from build123d import *

# Parameters (mm, degrees)
SKETCH_1_W           = 89.43
SKETCH_1_H           = 60
EXTRUDE_2_DEPTH      = 50
EXTRUDE_START        = -50
EXTRUDE_3_OUTLINE_W  = 85.42
EXTRUDE_3_OUTLINE_H  = 56
EXTRUDE_3_DEPTH      = 50
SKETCH_3_W           = 89.43
SKETCH_3_H           = 60
EXTRUDE_4_DEPTH      = 2
EXTRUDE_START_2      = -2
EXTRUDE_5_OUTLINE_W  = 73.44
EXTRUDE_5_OUTLINE_H  = 48.96
EXTRUDE_5_DEPTH      = 2
SKETCH_6_W           = 2
SKETCH_6_H           = 12
CUT_EXTRUDE_6_DEPTH  = 10
SKETCH_8_W           = 6
SKETCH_8_H           = 16
CUT_EXTRUDE_7_DEPTH  = 10
DRAFT_2_ANGLE        = 45
SKETCH_9_W           = 61
SKETCH_9_H           = 3
EXTRUDE_5_2_DEPTH    = 7
SKETCH_10_W          = 3
SKETCH_10_H          = 40
EXTRUDE_6_DEPTH      = 7
SKETCH_11_W          = 8
SKETCH_11_H          = 2
EXTRUDE_7_DEPTH      = 20
SKETCH_12_W          = 3
SKETCH_12_H          = 7
CUT_EXTRUDE_8_DEPTH  = 6
SKETCH_13_W          = 8
SKETCH_13_H          = 2
EXTRUDE_8_DEPTH      = 11
SKETCH_14_W          = 3
SKETCH_14_H          = 56
CUT_EXTRUDE_10_DEPTH = 11
SKETCH_15_W          = 87.425
SKETCH_15_H          = 2
CUT_EXTRUDE_11_DEPTH = 1
SKETCH_16_W          = 87.425
SKETCH_16_H          = 2
CUT_EXTRUDE_12_DEPTH = 1
SKETCH_17_R          = 3
CUT_EXTRUDE_13_DEPTH = 5.4
EXTRUDE_9_DEPTH      = 3.6
SKETCH_20_W          = 3
SKETCH_20_H          = 2
EXTRUDE_10_DEPTH     = 7
CUT_EXTRUDE_15_DEPTH = 7
SKETCH_22_W          = 32
SKETCH_22_H          = 58
CUT_EXTRUDE_16_DEPTH = 1
SKETCH_25_W          = 3
SKETCH_25_H          = 2
CUT_EXTRUDE_18_DEPTH = 2
SKETCH_27_W          = 4
SKETCH_27_H          = 2
CUT_EXTRUDE_19_DEPTH = 2
SKETCH_29_W          = 2.005
SKETCH_29_H          = 11.917011913
EXTRUDE_12_DEPTH     = 17
SKETCH_31_W          = 1.611039623
SKETCH_31_H          = 56
SKETCH_31_W_2        = 2
CUT_EXTRUDE_20_DEPTH = 48
SKETCH_34_W          = 8.005
SKETCH_34_H          = 34
EXTRUDE_13_DEPTH     = 2
SKETCH_35_W          = 8.005
SKETCH_35_H          = 3
EXTRUDE_14_DEPTH     = 8
SKETCH_36_R          = 3
CUT_EXTRUDE_21_DEPTH = 8
SKETCH_37_W          = 4
SKETCH_37_H          = 2
CUT_EXTRUDE_22_DEPTH = 5
SKETCH_38_W          = 10
SKETCH_38_H          = 3
CUT_EXTRUDE_23_DEPTH = 4.5
SKETCH_39_W          = 1.5
SKETCH_39_H          = 5
CUT_EXTRUDE_24_DEPTH = 20


# Read off the part's stored shape, not the designer's step: 切除-拉伸3, 切除-拉伸5
with BuildPart() as part:
    # 草图1 → 凸台-拉伸2 (new body)
    with BuildSketch(Plane.XY):
        Rectangle(SKETCH_1_W, SKETCH_1_H)
    extrude(amount=EXTRUDE_2_DEPTH)

    # 切除-拉伸3 outline → 切除-拉伸3 (cut)
    with BuildSketch(Plane.XY.offset(50).offset(EXTRUDE_START)):
        Rectangle(EXTRUDE_3_OUTLINE_W, EXTRUDE_3_OUTLINE_H)
    extrude(amount=EXTRUDE_3_DEPTH, mode=Mode.SUBTRACT)

    # 草图3 → 凸台-拉伸4 (add)
    with BuildSketch(Plane.XY.offset(50)):
        Rectangle(SKETCH_3_W, SKETCH_3_H)
    extrude(amount=-EXTRUDE_4_DEPTH)

    # Extrude 5 outline → Extrude 5 (cut)
    with BuildSketch(Plane.XY.offset(50).offset(EXTRUDE_START_2)):
        with Locations((-2.475, 0)):
            Rectangle(EXTRUDE_5_OUTLINE_W, EXTRUDE_5_OUTLINE_H)
    extrude(amount=EXTRUDE_5_DEPTH, mode=Mode.SUBTRACT)

    # 草图6 → 切除-拉伸6 (cut)
    with BuildSketch(Plane.ZY.offset(44.715)):
        with Locations((26.25, 14.9)):
            Rectangle(SKETCH_6_W, SKETCH_6_H)
    extrude(amount=-CUT_EXTRUDE_6_DEPTH, mode=Mode.SUBTRACT)

    # 草图8 → 切除-拉伸7 (cut)
    with BuildSketch(Plane.ZY.offset(44.715)):
        with Locations((26.25, 14.9)):
            Rectangle(SKETCH_8_W, SKETCH_8_H)
    extrude(amount=-CUT_EXTRUDE_7_DEPTH, mode=Mode.SUBTRACT)

    # 拔模2
    draft_2_faces = [part.faces().sort_by_distance(p)[0] for p in [
        (-43.7125, 22.9, 26.25),
        (-43.7125, 14.9, 23.25),
        (-43.7125, 6.9, 26.25),
        (-43.7125, 14.9, 29.25),
    ]]
    draft(draft_2_faces, Plane(origin=(-44.715, 30, 50), x_dir=(0, -1, 0), z_dir=(-1, 0, 0)), DRAFT_2_ANGLE)

    # 草图9 → Extrude 5 2 (add)
    with BuildSketch(Plane(origin=(0, -28, 0), x_dir=(1, 0, 0), z_dir=(0, 1, 0))):
        with Locations((-12.21, -38.5)):
            Rectangle(SKETCH_9_W, SKETCH_9_H)
    extrude(amount=EXTRUDE_5_2_DEPTH)

    # 草图10 → 凸台-拉伸6 (add)
    with BuildSketch(Plane(origin=(0, -28, 0), x_dir=(1, 0, 0), z_dir=(0, 1, 0))):
        with Locations((16.79, -20)):
            Rectangle(SKETCH_10_W, SKETCH_10_H)
    extrude(amount=EXTRUDE_6_DEPTH)

    # 草图11 → 凸台-拉伸7 (add)
    with BuildSketch(Plane(origin=(0, 0, 37), x_dir=(-1, 0, 0), z_dir=(0, 0, -1))):
        with Locations((-11.29, -22)):
            Rectangle(SKETCH_11_W, SKETCH_11_H)
        with Locations((38.71, -22)):
            Rectangle(SKETCH_11_W, SKETCH_11_H)
    extrude(amount=EXTRUDE_7_DEPTH)

    # 草图12 → 切除-拉伸8 (cut)
    with BuildSketch(Plane(origin=(0, 0, 0), x_dir=(-1, 0, 0), z_dir=(0, 0, -1))):
        with Locations((-16.79, -24.5)):
            Rectangle(SKETCH_12_W, SKETCH_12_H)
    extrude(amount=-CUT_EXTRUDE_8_DEPTH, mode=Mode.SUBTRACT)

    # 草图13 → 凸台-拉伸8 (add)
    with BuildSketch(Plane(origin=(0, 0, 17), x_dir=(-1, 0, 0), z_dir=(0, 0, -1))):
        with Locations((-11.29, -22)):
            Rectangle(SKETCH_13_W, SKETCH_13_H)
        with Locations((38.71, -22)):
            Rectangle(SKETCH_13_W, SKETCH_13_H)
    extrude(amount=EXTRUDE_8_DEPTH)

    # 草图14 → 切除-拉伸10 (cut)
    with BuildSketch(Plane(origin=(44.715, 0, 0), x_dir=(0, 0, -1), z_dir=(1, 0, 0))):
        with Locations((-1.5, 0)):
            Rectangle(SKETCH_14_W, SKETCH_14_H)
    extrude(amount=-CUT_EXTRUDE_10_DEPTH, mode=Mode.SUBTRACT)

    # 草图15 → 切除-拉伸11 (cut)
    with BuildSketch(Plane.XZ.offset(-28)):
        with Locations((1.0025, 2)):
            Rectangle(SKETCH_15_W, SKETCH_15_H)
    extrude(amount=-CUT_EXTRUDE_11_DEPTH, mode=Mode.SUBTRACT)

    # 草图16 → 切除-拉伸12 (cut)
    with BuildSketch(Plane(origin=(0, -28, 0), x_dir=(1, 0, 0), z_dir=(0, 1, 0))):
        with Locations((1.0025, -2)):
            Rectangle(SKETCH_16_W, SKETCH_16_H)
    extrude(amount=-CUT_EXTRUDE_12_DEPTH, mode=Mode.SUBTRACT)

    # 草图17 → 切除-拉伸13 (cut)
    with BuildSketch(Plane.ZY.offset(44.715)):
        with Locations(Location((11.4, 18, 0), (0, 0, 270))):
            Circle(SKETCH_17_R)
    extrude(amount=-CUT_EXTRUDE_13_DEPTH, mode=Mode.SUBTRACT)

    # 草图18 → 凸台-拉伸9 (add)
    with BuildSketch(Plane(origin=(0, -28, 0), x_dir=(1, 0, 0), z_dir=(0, 1, 0))):
        Polygon((18.29, -25), (18.29, -27), (40.29, -27), (40.29, -18), (38.29, -18), (38.29, -25), align=None)
    extrude(amount=EXTRUDE_9_DEPTH)

    # 草图20 → 凸台-拉伸10 (add)
    with BuildSketch(Plane(origin=(0, 0, 25), x_dir=(-1, 0, 0), z_dir=(0, 0, -1))):
        with Locations((-36.79, -25.4)):
            Rectangle(SKETCH_20_W, SKETCH_20_H)
        with Locations((-19.79, -25.4)):
            Rectangle(SKETCH_20_W, SKETCH_20_H)
    extrude(amount=EXTRUDE_10_DEPTH)

    # 草图21 → 切除-拉伸15 (cut)
    with BuildSketch(Plane(origin=(0, -28, 0), x_dir=(1, 0, 0), z_dir=(0, 1, 0))):
        with BuildLine():
            Line((25.28, -20), (31.3, -20))
            ThreePointArc((31.3, -20), (32.353589104, -20.436410896), (32.79, -21.49))
            Line((32.79, -21.49), (32.79, -21.51))
            ThreePointArc((32.79, -21.51), (32.353589104, -22.563589104), (31.3, -23))
            Line((31.3, -23), (25.28, -23))
            ThreePointArc((25.28, -23), (24.226410896, -22.563589104), (23.79, -21.51))
            Line((23.79, -21.51), (23.79, -21.49))
            ThreePointArc((23.79, -21.49), (24.226410896, -20.436410896), (25.28, -20))
        make_face()
    extrude(amount=-CUT_EXTRUDE_15_DEPTH, mode=Mode.SUBTRACT)

    # 草图22 → 切除-拉伸16 (cut)
    with BuildSketch(Plane(origin=(0, 0, 0), x_dir=(-1, 0, 0), z_dir=(0, 0, -1))):
        with Locations((-28.715, 0)):
            Rectangle(SKETCH_22_W, SKETCH_22_H)
    extrude(amount=-CUT_EXTRUDE_16_DEPTH, mode=Mode.SUBTRACT)

    # 草图25 → 切除-拉伸18 (cut)
    with BuildSketch(Plane(origin=(0, -21, 0), x_dir=(1, 0, 0), z_dir=(0, 1, 0))):
        with Locations((16.79, -39)):
            Rectangle(SKETCH_25_W, SKETCH_25_H)
    extrude(amount=-CUT_EXTRUDE_18_DEPTH, mode=Mode.SUBTRACT)

    # 草图27 → 切除-拉伸19 (cut)
    with BuildSketch(Plane(origin=(0, -21, 0), x_dir=(1, 0, 0), z_dir=(0, 1, 0))):
        with Locations((16.29, -39)):
            Rectangle(SKETCH_27_W, SKETCH_27_H)
    extrude(amount=-CUT_EXTRUDE_19_DEPTH, mode=Mode.SUBTRACT)

    # 草图29 → 凸台-拉伸12 (add)
    with BuildSketch(Plane(origin=(0, 0, 0), x_dir=(-1, 0, 0), z_dir=(0, 0, -1))):
        with Locations((43.7125, 17.342942197)):
            Rectangle(SKETCH_29_W, SKETCH_29_H)
    extrude(amount=-EXTRUDE_12_DEPTH)

    # 草图31 → 切除-拉伸20 (cut)
    with BuildSketch(Plane(origin=(0, 0, 0), x_dir=(-1, 0, 0), z_dir=(0, 0, -1))):
        with Locations((-41.909480188, 0)):
            Rectangle(SKETCH_31_W, SKETCH_31_H)
        with Locations((41.715, 0)):
            Rectangle(SKETCH_31_W_2, SKETCH_31_H)
    extrude(amount=-CUT_EXTRUDE_20_DEPTH, mode=Mode.SUBTRACT)

    # 草图34 → 凸台-拉伸13 (add)
    with BuildSketch(Plane(origin=(0, -21, 0), x_dir=(1, 0, 0), z_dir=(0, 1, 0))):
        with Locations((-38.7125, -23)):
            Rectangle(SKETCH_34_W, SKETCH_34_H)
    extrude(amount=-EXTRUDE_13_DEPTH)

    # 草图35 → 凸台-拉伸14 (add)
    with BuildSketch(Plane(origin=(0, -21, 0), x_dir=(1, 0, 0), z_dir=(0, 1, 0))):
        with Locations((-38.7125, -38.5)):
            Rectangle(SKETCH_35_W, SKETCH_35_H)
    extrude(amount=-EXTRUDE_14_DEPTH)

    # 草图36 → 切除-拉伸21 (cut)
    with BuildSketch(Plane(origin=(-42.715, 0, 0), x_dir=(0, 0, -1), z_dir=(1, 0, 0))):
        with Locations(Location((-5.6, 14.8, 0), (0, 0, 90))):
            Circle(SKETCH_36_R)
    extrude(amount=-CUT_EXTRUDE_21_DEPTH, mode=Mode.SUBTRACT)

    # 草图37 → 切除-拉伸22 (cut)
    with BuildSketch(Plane(origin=(0, -23, 0), x_dir=(1, 0, 0), z_dir=(0, 1, 0))):
        with Locations((16.29, -39)):
            Rectangle(SKETCH_37_W, SKETCH_37_H)
    extrude(amount=-CUT_EXTRUDE_22_DEPTH, mode=Mode.SUBTRACT)

    # 草图38 → 切除-拉伸23 (cut)
    with BuildSketch(Plane.XY.offset(40)):
        with Locations((-30.715, -22.5)):
            Rectangle(SKETCH_38_W, SKETCH_38_H)
    extrude(amount=-CUT_EXTRUDE_23_DEPTH, mode=Mode.SUBTRACT)

    # 草图39 → 切除-拉伸24 (cut)
    with BuildSketch(Plane(origin=(0, 0, 6), x_dir=(-1, 0, 0), z_dir=(0, 0, -1))):
        with Locations((-16.04, -25.5)):
            Rectangle(SKETCH_39_W, SKETCH_39_H)
    extrude(amount=-CUT_EXTRUDE_24_DEPTH, mode=Mode.SUBTRACT)


solid = part.part
Read the model definition and answer for the solid it produces. Units are mm, in the model's axes. A direction names the side the tool comes from. Give positions to 0.01 mm unless a question says otherwise; leave off trailing zeros. Loops run counter-clockwise (first coordinate to the right, second up) from the corner with the lowest first, then second, coordinate; pieces in that order, holes last. Notation, with made-up numbers: (-21.5, 7.25) -> (24.5, 7.25) arc R19 cw to (24.5, 18.25) -> close; hole circle Ø4 at (54, -30.75). An arc over 180 degrees is marked (long way). Use a Markdown table: item, result.
Q1. Determine the mould class of faces 4 (the face through (32, -24.4, 26)), 5 (the face through (-3, -24.48, 49)), 6 (the face through (-1, -26, 50)), 7 (the face through (-43.729, 14.788, 24.236)) for opening direction X: pulls with the +X half, pulls with the -X half, needs draft (parallel to the pull), parting line crosses it, or undercut.
Solved:
| item | result |
|---|---|
| face 4 | undercut |
| face 5 | undercut |
| face 6 | needs draft |
| face 7 | pulls with the -X half |
Q2. Section A-A, the plane y = 14.8 is taken. Determine the outline of the cut face in (x, z) (3 decimals).
Solved:
| item | result |
|---|---|
| outline | (-44.715, 0) -> (-42.715, 0) -> (-42.715, 2.6) -> (-44.715, 2.6) -> close; (-44.715, 8.6) -> (-42.715, 8.6) -> (-42.715, 25.25) -> (-44.715, 23.25) -> close; (-44.715, 29.25) -> (-42.715, 27.25) -> (-42.715, 48) -> (-39.195, 48) -> (-39.195, 50) -> (-44.715, 50) -> close; (34.245, 48) -> (42.715, 48) -> (42.715, 3) -> (44.715, 3) -> (44.715, 50) -> (34.245, 50) -> close |
Q3. Each of these flat-tipped pins is pushed along its axis until it touches: pin 1 (3 mm diameter, centred on x = 32.5, y = -26, fed in from -Z); pin 2 (12 mm diameter, centred on x = -19.5, y = -11.5, fed in from +Z); pin 3 (1.5 mm diameter, centred on x = 15.5, y = -23, fed in from +Z). Where does it stop, or does it pass through?
Solved:
| item | result |
|---|---|
| pin 1 | stops at z = 25 |
| pin 2 | passes through |
| pin 3 | stops at z = 38 |
Q4. Section B-B, the plane z = 32.5 is taken. Determine the outline of the cut face in (x, y) (3 decimals).
Solved:
| item | result |
|---|---|
| outline | (-44.715, -30) -> (44.715, -30) -> (44.715, 30) -> (-44.715, 30) -> close; hole (-42.715, -28) -> (15.29, -28) -> (15.29, -23) -> (7.29, -23) -> (7.29, -21) -> (18.29, -21) -> (18.29, -28) -> (42.715, -28) -> (42.715, 28) -> (-42.715, 28) -> (-42.715, -21) -> (-34.71, -21) -> (-34.71, -23) -> (-42.715, -23) -> close |
Q5. Section C-C, the plane x = 3.5 is taken. Determine the outline of the cut face in (y, z), then the cut area to 3 significant figures.
Solved:
| item | result |
|---|---|
| outline | (-30, 0) -> (-28, 0) -> (-28, 1) -> (-29, 1) -> (-29, 3) -> (-28, 3) -> (-28, 37) -> (-21, 37) -> (-21, 40) -> (-28, 40) -> (-28, 48) -> (-24.48, 48) -> (-24.48, 50) -> (-30, 50) -> close; (24.48, 48) -> (28, 48) -> (28, 3) -> (29, 3) -> (29, 1) -> (28, 1) -> (28, 0) -> (30, 0) -> (30, 50) -> (24.48, 50) -> close |
| area | 231 mm^2 |
Q6. Section D-D, the plane y = 0 is taken. Determine the outline of the cut face in (x, z) (3 decimals), then the cut area to 3 significant figures.
Solved:
| item | result |
|---|---|
| outline | (-44.715, 0) -> (-42.715, 0) -> (-42.715, 48) -> (-39.195, 48) -> (-39.195, 50) -> (-44.715, 50) -> close; (34.245, 48) -> (42.715, 48) -> (42.715, 3) -> (44.715, 3) -> (44.715, 50) -> (34.245, 50) -> close |
| area | 218 mm^2 |
Q7. A tool of negligible diameter and unlimited length cuts with its end or side. For faces 1 (the face through (21.29, -25, 22)), 2 (the face through (-43.7, 17.57, 4.45)), 3 (the face through (28, -29, 20)), from which of +Z, -Z, +X, -X, +Y, -Y can it reach the whole face along a straight path? Write none if from no direction.
Solved:
| item | result |
|---|---|
| face 1 | -Z |
| face 2 | -X |
| face 3 | -Y |
Q8. Find the intervals of material crossed by line 1 along Y through (x, z) = (-41, 16); line 2 along X through (y, z) = (12, 31) (3 decimals); line 3 along X through (y, z) = (-25, 35.5) (3 decimals), in increasing order.
Solved:
| item | result |
|---|---|
| line 1 | y = -30 to -28, -23 to -21, 28 to 30 |
| line 2 | x = -44.715 to -42.715, 42.715 to 44.715 |
| line 3 | x = -44.715 to -42.715, 15.29 to 18.29, 42.715 to 44.715 |
